Read the model definition and answer for the solid it produces. Units are mm, in the model's axes. Coordinates: 2 decimals unless noted, no trailing zeros. Order: outer loops, then holes, each group sorted by start corner. A loop starts at its lowest first (then second) coordinate and runs counter-clockwise, first axis right, second up. Notation, with made-up numbers: (7, -30) - (14, -30) arc R15 ccw to (14, -4) - close; hole circle Ø5 at (49, 44). An arc over 180 degrees is marked (long way). Answer as a JSON object with one key per item and string values. Group by question number.
from build123d import *

# Parameters (mm, degrees)
F1_DEPTH = 200
F2_R     = 1


with BuildPart() as f1:
    # F0 (on Right) → F1 (new body, symmetric)
    with BuildSketch(Plane.YZ):
        Polygon((-12, 8), (-12, 0), (0, 0), (0, 272), (-12, 272), (-12, 20.5), (-8, 20.5), (-8, 8), align=None)
    extrude(amount=F1_DEPTH, both=True)

    # F2
    f2_edges = [f1.edges().sort_by_distance(p)[0] for p in [
        (-200, -6, 272),
        (200, -6, 272),
        (200, -6, 0),
        (-200, -6, 0),
    ]]
    fillet(f2_edges, radius=F2_R)


solid = f1.part
1. A straight line is drawn through the part: L1, parallel to Z at x = 31.5, y = -8.5. Find the intervals that lie inside material, in ascending order.
2. Given pin 1 (4 mm diameter, centred on x = 71, z = 17, fed in from -Y), flat-ended and moving along its own axis, determine where the tip first touches the part or whether it passes through.
3. For a pull along Z with two mould halves and no side action, classify faces 1 (the flat face through (3, -8, 14)), 2 (the flat face through (3, -6, 0)), 3 (the flat face through (200, -6, 138)) as pulls with the +Z half, pulls with the -Z half, needs draft (parallel to the pull), parting line crosses it, or undercut.
4. A cutting plane is placed at A-A on x = -134.5. Write down the section's boundary in (y, z), and give its area (3 significant figures).
Derived:
{
 "1": {"L1": "z = 0 to 8, 20.5 to 272"},
 "2": {"pin 1": "stops at y = -8"},
 "3": {"face 1": "undercut", "face 2": "pulls with the -Z half", "face 3": "needs draft"},
 "4": {"outline": "(-12, 0) - (0, 0) - (0, 272) - (-12, 272) - (-12, 20.5) - (-8, 20.5) - (-8, 8) - (-12, 8) - close", "area": "3,210 mm2"}
}
